from build123d import *

# Parameters (mm, degrees)
SKETCH1_W           = 395
SKETCH1_H           = 250
BOSS_EXTRUDE1_DEPTH = 3
SKETCH2_W           = 75
SKETCH2_H           = 80
CUT_EXTRUDE1_DEPTH  = 3
SKETCH3_R           = 1.5
CUT_EXTRUDE2_DEPTH  = 10
FILLET1_R           = 5
LPATTERN1_COUNT     = 5
LPATTERN1_PITCH     = 10
LPATTERN1_COL_COUNT = 5
LPATTERN1_COL_PITCH = 10


with BuildPart() as part:
    # Sketch1 → Boss-Extrude1 (new body)
    with BuildSketch(Plane(origin=(0, 0, 0), x_dir=(1, 0, 0), z_dir=(0, 1, 0))):
        Rectangle(SKETCH1_W, SKETCH1_H)
    extrude(amount=BOSS_EXTRUDE1_DEPTH)

    # Sketch2 → Cut-Extrude1 (cut)
    with BuildSketch(Plane(origin=(0, 3, 0), x_dir=(1, 0, 0), z_dir=(0, 1, 0))):
        with Locations((-160, 85)):
            Rectangle(SKETCH2_W, SKETCH2_H)
    cut_extrude1 = extrude(amount=-CUT_EXTRUDE1_DEPTH, mode=Mode.SUBTRACT)

    # Mirror1: Cut-Extrude1 across plane
    add(cut_extrude1.mirror(Plane(origin=(0, 0, 0), x_dir=(0, 0, 1), z_dir=(1, 0, 0))), mode=Mode.SUBTRACT)

    # Sketch3 → Cut-Extrude2 (cut)
    with BuildSketch(Plane(origin=(0, 3, 0), x_dir=(1, 0, 0), z_dir=(0, 1, 0))):
        with Locations((0, -50)):
            Circle(SKETCH3_R)
        with Locations((0, -80)):
            Circle(SKETCH3_R)
    cut_extrude2 = extrude(amount=-CUT_EXTRUDE2_DEPTH, mode=Mode.SUBTRACT)

    # Fillet1
    fillet1_edges = [part.edges().sort_by_distance(p)[0] for p in [
        (-122.5, 1.5, -45),
        (122.5, 1.5, -45),
    ]]
    fillet(fillet1_edges, radius=FILLET1_R)

    # LPattern1: Cut-Extrude2 ×5
    with Locations(*[(-i * LPATTERN1_PITCH, 0, 0) for i in range(1, LPATTERN1_COUNT)]):
        add(cut_extrude2, mode=Mode.SUBTRACT)

    # LPattern1 col: Cut-Extrude2 ×5
    with Locations(*[(i * LPATTERN1_COL_PITCH, 0, 0) for i in range(1, LPATTERN1_COL_COUNT)]):
        add(cut_extrude2, mode=Mode.SUBTRACT)


solid = part.part
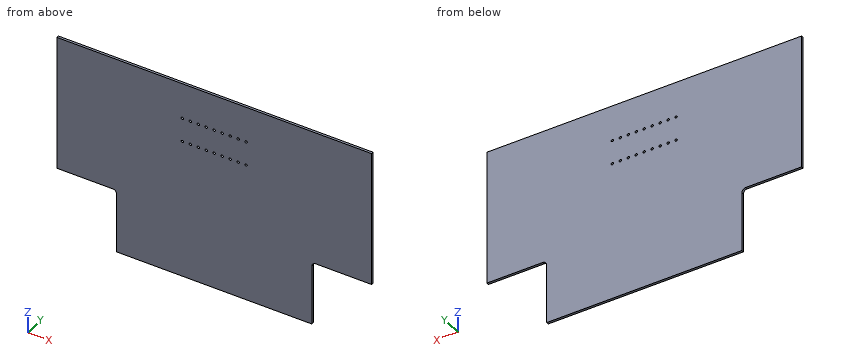
Read the model definition and answer for the solid it produces. Units are mm, in the model's axes. Give positions to 0.01 mm unless a question says otherwise; leave off trailing zeros. Loops run counter-clockwise (first coordinate to the right, second up) from the corner with the lowest first, then second, coordinate; pieces in that order, holes last. Notation, with made-up numbers: M -38.75,76.5 L -9.75,76.5 A22 cw -9.75,108.5 Z; hole C 79,74.5 d5. An arc over 180 degrees is marked long. Write each question's results on one line, items separated by ' | '.
1. Straight lines are drawn through the part: line 1 (Z direction, x = -30, y = 0.9); line 2 (Z direction, x = -132, y = 2.9); line 3 (X direction, y = 2.05, z = -67). For each, find the intervals that lie inside material, in ascending order. Write a range as [from, to].
Values:
line 1: z = [-125, 48.5], [51.5, 78.5], [81.5, 125] | line 2: z = [-45, 125] | line 3: x = [-122.5, 122.5]
2. Section A-A on y = 2.3 is taken. State how many separate pieces and enclosed holes the cut face has, plus the area to 3 significant figures.
Values:
separate pieces: 1 | enclosed holes: 18 | area: 86,600 mm^2
3. Section B-B on z = -105 is taken. Give the vertices of the cut face in (x, y), plus the area to 3 significant figures.
Values:
outline: M -122.5,0 L 122.5,0 L 122.5,3 L -122.5,3 Z | area: 735 mm^2
4. Given pin 1 (0.9 mm diameter, centred on y = 1.5, z = -84.5, fed in from -X); pin 2 (2.5 mm diameter, centred on x = 20, z = 50, fed in from -Y), each flat-ended and moving along its own axis, determine where each tip first touches the part or whether it passes through.
Values:
pin 1: stops at x = -122.5 | pin 2: passes through
